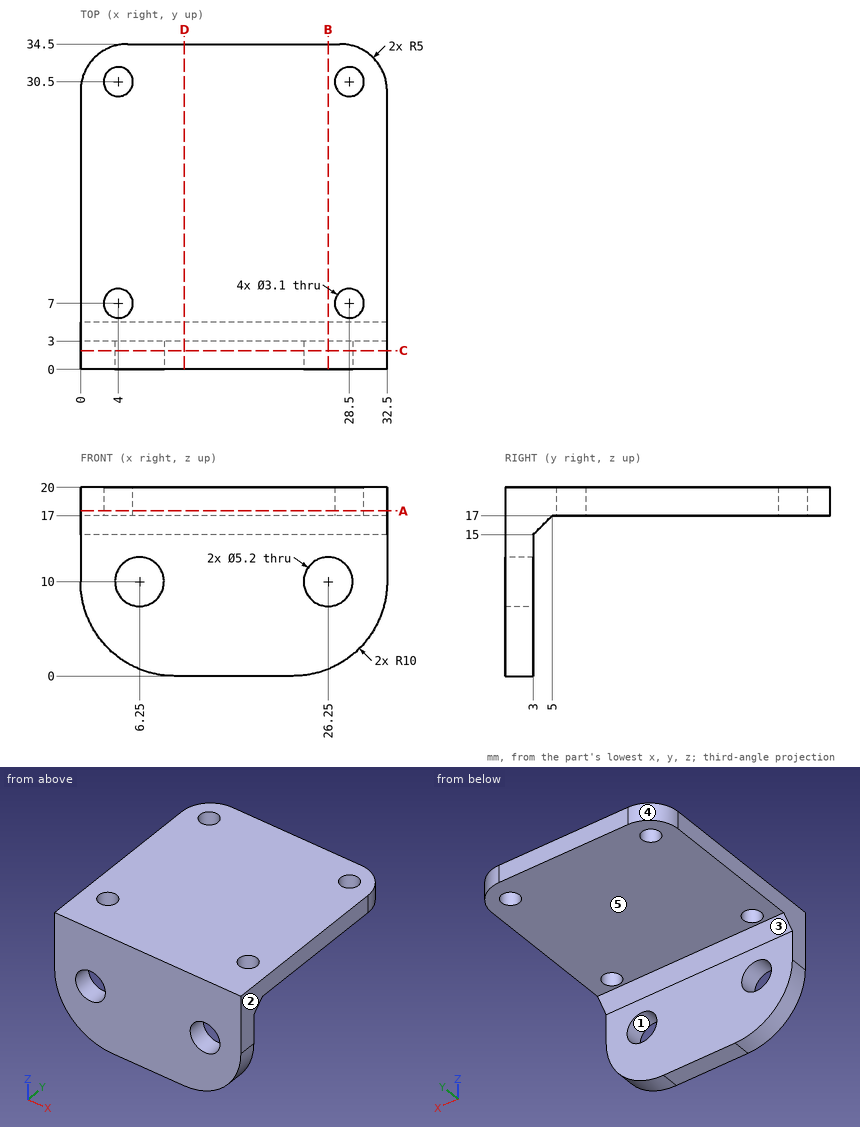
Geometry: see drawing. Coordinates: mm, zero at the bounding-box minimum. A direction names the side the tool comes from. Give positions to 0.01 mm unless a question says otherwise; leave off trailing zeros. Order: outer loops, then holes, each group sorted by start corner. A loop starts at its lowest first (then second) coordinate and runs counter-clockwise, first axis right, second up. Notation, with made-up numbers: (67.25, 87.5) - (122.25, 87.5) arc R15 cw to (122.25, 103.5) - close; hole circle Ø9 at (-9.5, 64). An arc over 180 degrees is marked (long way). Use a Markdown table: item, result.
(1) Pin query (flat end, axial travel): pin 1 (1 mm diameter, centred on x = 15, z = 7.5, fed in from +Y); pin 2 (3.5 mm diameter, centred on x = 28.5, y = 30.5, fed in from -Z); pin 3 (2.5 mm diameter, centred on x = 4, y = 30.5, fed in from +Z) (3 decimals). Return the tip coordinate at first contact, or that it passes through.
Computed values:
| item | result |
|---|---|
| pin 1 | stops at y = 3 |
| pin 2 | stops at z = 17 |
| pin 3 | passes through |
(2) Access query for the marked faces 4 and 5. Directions: +Z, -Z, +X, -X, +Y, -Y. A direction counts if a zero-diameter tool reaches every point of the face in a straight line with its end or side. Return the directions, or none.
Computed values:
| item | result |
|---|---|
| face 4 | +Z, -Z, -X, +Y |
| face 5 | -Z, +X, -X, +Y |
(3) Line query: line 1 (X direction, y = 2.1, z = 10); line 2 (Y direction, x = 4, z = 19.2); line 3 (Z direction, x = 15.5, y = 28.5). Output: solid intervals per line, ascending. Write a range as from..to.
Computed values:
| item | result |
|---|---|
| line 1 | x = 0..3.65, 8.85..23.65, 28.85..32.5 |
| line 2 | y = 0..5.45, 8.55..28.95, 32.05..34.4 |
| line 3 | z = 17..20 |
(4) Section query B-B (x = 26.25). Output: boundary loops of the cut face in (y, z).
Computed values:
| item | result |
|---|---|
| outline | (0, 0.73) - (3, 0.73) - (3, 7.4) - (0, 7.4) - close; (0, 12.6) - (3, 12.6) - (3, 15) - (5, 17) - (34.5, 17) - (34.5, 20) - (0, 20) - close |
(5) Section query A-A (z = 17.5). Output: boundary loops of the cut face in (x, y).
Computed values:
| item | result |
|---|---|
| outline | (0, 0) - (32.5, 0) - (32.5, 29.5) arc R5 ccw to (27.5, 34.5) - (5, 34.5) arc R5 ccw to (0, 29.5) - close; hole circle Ø3.1 at (4, 7); hole circle Ø3.1 at (4, 30.5); hole circle Ø3.1 at (28.5, 7); hole circle Ø3.1 at (28.5, 30.5) |
(6) Section query C-C (y = 2). Output: boundary loops of the cut face in (x, z).
Computed values:
| item | result |
|---|---|
| outline | (0, 10) arc R10 ccw to (10, 0) - (22.5, 0) arc R10 ccw to (32.5, 10) - (32.5, 20) - (0, 20) - close; hole circle Ø5.2 at (6.25, 10); hole circle Ø5.2 at (26.25, 10) |
(7) Section query D-D (x = 11). Output: boundary loops of the cut face in (y, z).
Computed values:
| item | result |
|---|---|
| outline | (0, 0) - (3, 0) - (3, 15) - (5, 17) - (34.5, 17) - (34.5, 20) - (0, 20) - close |
(8) Draft query along Z for the marked faces 1, 2 and 3. Return one class per face: released by +Z, released by -Z, zero draft, split by the parting line, or undercut.
Computed values:
| item | result |
|---|---|
| face 1 | undercut |
| face 2 | zero draft |
| face 3 | released by -Z |
